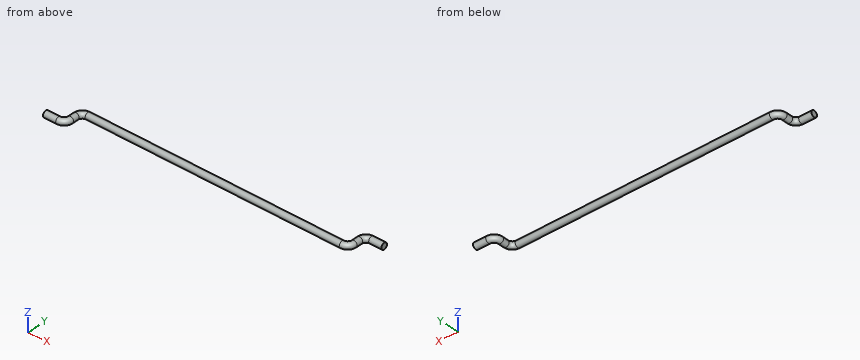
Autodesk Inventor part; units mm, degrees
ref_plane "YZ Plane" through (0, 0, 0) normal (1, 0, 0) x (0, 1, 0)
ref_plane "XZ Plane" through (0, 0, 0) normal (0, 1, 0) x (-1, 0, 0)
ref_plane "XY Plane" through (0, 0, 0) normal (0, 0, 1) x (1, 0, 0)
sketch "Skizze1" plane through (0, 0, 0) normal (0, 0, 1) x (1, 0, 0)
  line L0 (0, 0) -> (2, 0)
  line L1 (3, 1) -> (3, 2)
  line L2 (4, 3) -> (44, 3)
  line L3 (45, 4) -> (45, 5)
  line L4 (46, 6) -> (48, 6)
  arc A0 (2, 0) -> (3, 1) centre (2, 1) ccw
  arc A1 (4, 3) -> (3, 2) centre (4, 2) ccw
  arc A2 (44, 3) -> (45, 4) centre (44, 4) ccw
  arc A3 (46, 6) -> (45, 5) centre (46, 5) ccw
  dimension "d0" = 1
  dimension "d4" = 2
  dimension "d5" = 3
  dimension "d6" = 3
  dimension "d7" = 40
  dimension "d8" = 2
sketch "Skizze2" plane through (0, 0, 0) normal (1, 0, 0) x (0, 1, 0)
  circle A0 centre (0, 0) radius 0.5
  dimension "d1" = 1
sweep "Sweeping1" add profiles "Skizze2" path "Skizze1"
properties part number "P_Wing_mid_servolink"
Part model, mm, in its own coordinate system. Round coordinates to 2 decimals unless told otherwise and drop trailing zeros. Order: outer loops, then holes, each group sorted by start corner. A loop starts at its lowest first (then second) coordinate and runs counter-clockwise, first axis right, second up. Notation, with made-up numbers: M -33.5,45.25 L -27.5,45.25 A7 ccw -27.5,51.25 Z; hole C 83,-2.5 d5. An arc over 180 degrees is marked long. Answer in a Markdown table with one row per item. Add a question column.
Q1. Cut at B-B on x = 41. Give the cut face in (y, z), and give its area (3 significant figures).
Q2. Cut at A-A on z = 0. Give the cut face in (x, y).
Q3. Wall check: L1, parallel to X at y = 1, z = 0.1; L2, parallel to X at y = 2.5, z = -0.35. Give the ranges that are in metal, low to high. Write a range as from..to.
Established:
| question | item | result |
|---|---|---|
| 1 | outline | C 3,0 d1 |
| 1 | area | 0.785 mm2 |
| 2 | outline | M 0,-0.5 L 2,-0.5 A1.5 ccw 3.5,1 L 3.5,2 A0.5 cw 4,2.5 L 44,2.5 A1.5 ccw 45.5,4 L 45.5,5 A0.5 cw 46,5.5 L 48,5.5 L 48,6.5 L 46,6.5 A1.5 ccw 44.5,5 L 44.5,4 A0.5 cw 44,3.5 L 4,3.5 A1.5 ccw 2.5,2 L 2.5,1 A0.5 cw 2,0.5 L 0,0.5 Z |
| 3 | L1 | x = 2.51..3.49 |
| 3 | L2 | x = 2.74..3.6 |
